Could you check a few things on this model? Use its own coordinates, in mm. A direction names the side the tool comes from. Round coordinates to 2 decimals unless told otherwise and drop trailing zeros. Loops run counter-clockwise (first coordinate to the right, second up) from the corner with the lowest first, then second, coordinate; pieces in that order, holes last. Notation, with made-up numbers: M 7,-11 L 19,-11 A9 ccw 19,6 Z; hole C -15.75,52.25 d1. An arc over 180 degrees is marked long. Answer in a Markdown table with one row per item.
```python
from build123d import *

# Parameters (mm, degrees)
BOSS_EXTRUDE1_DEPTH                 = 7
SKETCH3_W                           = 68
SKETCH3_H                           = 66
BOSS_EXTRUDE2_DEPTH                 = 7
SKETCH5_R                           = 1
HOLE_POSITIONS_DEPTH                = 74.137994469
M5X0_8_TAPPED_HOLE1_D               = 4.2
CBORE_FOR_M3_SHCS1_D                = 3.4
CBORE_FOR_M3_SHCS1_CBORE_D          = 7
CBORE_FOR_M3_SHCS1_CBORE_DEPTH      = 3
FILLET1_R                           = 8
FILLET2_R                           = 4
M3X0_5_TAPPED_HOLE1_D               = 2.5
M3X0_5_TAPPED_HOLE1_DEPTH           = 7.5
M3X0_5_TAPPED_HOLE1_TIP             = 0.751075774
M3X0_5_TAPPED_HOLE1_ON_FACE_2_D     = 2.5
M3X0_5_TAPPED_HOLE1_ON_FACE_2_DEPTH = 7.5
M3X0_5_TAPPED_HOLE1_ON_FACE_2_TIP   = 0.751075774
M3X0_5_TAPPED_HOLE1_ON_FACE_3_D     = 2.5
M3X0_5_TAPPED_HOLE1_ON_FACE_3_DEPTH = 7.5
M3X0_5_TAPPED_HOLE1_ON_FACE_3_TIP   = 0.751075774
CHAMFER1_SIZE                       = 0.8


with BuildPart() as part:
    # Sketch1 → Boss-Extrude1 (new body)
    with BuildSketch(Plane(origin=(0, 0, 0), x_dir=(1, 0, 0), z_dir=(0, 1, 0))):
        Polygon((0, -55.033320997), (47.660254038, 27.516660498), (-47.660254038, 27.516660498), align=None)
    extrude(amount=BOSS_EXTRUDE1_DEPTH)

    # Sketch3 → Boss-Extrude2 (add)
    with BuildSketch(Plane(origin=(0, 0, 0), x_dir=(1, 0, 0), z_dir=(0, 1, 0))):
        with Locations((0, -5.483339502)):
            Rectangle(SKETCH3_W, SKETCH3_H)
    extrude(amount=BOSS_EXTRUDE2_DEPTH)

    # Sketch5 → Hole Positions (cut, through all)
    with BuildSketch(Plane(origin=(0, 7, 0), x_dir=(1, 0, 0), z_dir=(0, 1, 0))):
        with Locations(Location((-34, 19.629909152, 0), (0, 0, 270))):
            Circle(SKETCH5_R)
        with Locations(Location((34, 19.629909152, 0), (0, 0, 270))):
            Circle(SKETCH5_R)
        with Locations(Location((0, -39.259818305, 0), (0, 0, 270))):
            Circle(SKETCH5_R)
    extrude(amount=-HOLE_POSITIONS_DEPTH, mode=Mode.SUBTRACT)

    # M5x0.8 Tapped Hole1 (through all)
    with Locations(Plane(origin=(0, 7, 0), x_dir=(1, 0, 0), z_dir=(0, 1, 0))):
        with Locations((-34, 19.629909152), (34, 19.629909152), (0, -39.259818305)):
            Hole(M5X0_8_TAPPED_HOLE1_D / 2)

    # CBORE for M3 SHCS1 (through all)
    with Locations(Plane(origin=(0, 7, 0), x_dir=(1, 0, 0), z_dir=(0, 1, 0))):
        with Locations((-10, 2), (10, 2), (10, -18), (-10, -18)):
            CounterBoreHole(CBORE_FOR_M3_SHCS1_D / 2, CBORE_FOR_M3_SHCS1_CBORE_D / 2, CBORE_FOR_M3_SHCS1_CBORE_DEPTH)

    # Fillet1
    fillet1_edges = [part.edges().sort_by_distance(p)[0] for p in [
        (-47.660254038, 3.5, -27.516660498),
        (47.660254038, 3.5, -27.516660498),
        (0, 3.5, 55.033320997),
    ]]
    fillet(fillet1_edges, radius=FILLET1_R)

    # Fillet2
    fillet2_edges = [part.edges().sort_by_distance(p)[0] for p in [
        (34, 3.5, -3.856406461),
        (34, 3.5, 38.483339502),
        (-34, 3.5, -3.856406461),
        (-9.555136271, 3.5, 38.483339502),
        (-34, 3.5, 38.483339502),
        (9.555136271, 3.5, 38.483339502),
    ]]
    fillet(fillet2_edges, radius=FILLET2_R)

    # M3x0.5 Tapped Hole1
    with Locations(Plane(origin=(-34, 3.5, 28.483339502), x_dir=(0, 0, -1), z_dir=(-1, 0, 0))):
        with Locations((0, 0)):
            Hole(M3X0_5_TAPPED_HOLE1_D / 2, depth=M3X0_5_TAPPED_HOLE1_DEPTH)
            with Locations((0, 0, -(M3X0_5_TAPPED_HOLE1_DEPTH + M3X0_5_TAPPED_HOLE1_TIP / 2))):  # 118° drill point
                Cone(0, M3X0_5_TAPPED_HOLE1_D / 2, M3X0_5_TAPPED_HOLE1_TIP, mode=Mode.SUBTRACT)

    # M3x0.5 Tapped Hole1 on face 2
    with Locations(Plane(origin=(34, 3.5, 28.483339502), x_dir=(0, 0, 1), z_dir=(1, 0, 0))):
        with Locations((0, 0)):
            Hole(M3X0_5_TAPPED_HOLE1_ON_FACE_2_D / 2, depth=M3X0_5_TAPPED_HOLE1_ON_FACE_2_DEPTH)
            with Locations((0, 0, -(M3X0_5_TAPPED_HOLE1_ON_FACE_2_DEPTH + M3X0_5_TAPPED_HOLE1_ON_FACE_2_TIP / 2))):  # 118° drill point
                Cone(0, M3X0_5_TAPPED_HOLE1_ON_FACE_2_D / 2, M3X0_5_TAPPED_HOLE1_ON_FACE_2_TIP, mode=Mode.SUBTRACT)

    # M3x0.5 Tapped Hole1 on face 3
    with Locations(Plane(origin=(0, 3.5, -27.516660498), x_dir=(-1, 0, 0), z_dir=(0, 0, -1))):
        with Locations((0, 0)):
            Hole(M3X0_5_TAPPED_HOLE1_ON_FACE_3_D / 2, depth=M3X0_5_TAPPED_HOLE1_ON_FACE_3_DEPTH)
            with Locations((0, 0, -(M3X0_5_TAPPED_HOLE1_ON_FACE_3_DEPTH + M3X0_5_TAPPED_HOLE1_ON_FACE_3_TIP / 2))):  # 118° drill point
                Cone(0, M3X0_5_TAPPED_HOLE1_ON_FACE_3_D / 2, M3X0_5_TAPPED_HOLE1_ON_FACE_3_TIP, mode=Mode.SUBTRACT)

    # Chamfer1
    chamfer1_edges = [part.edges().sort_by_distance(p)[0] for p in [
        (-13.5, 7, -2),
        (-8.3, 0, -2),
        (0, 7, -27.516660498),
        (0, 0, -27.516660498),
        (-37.633974596, 0, -10.150635095),
        (7.664319482, 0, 41.758330249),
        (0, 0, 47.033320997),
        (-40.732050808, 0, -23.516660498),
        (40.732050808, 0, -23.516660498),
        (7.664319482, 7, 41.758330249),
        (-37.633974596, 7, -10.150635095),
        (0, 7, 47.033320997),
        (-40.732050808, 7, -23.516660498),
        (40.732050808, 7, -23.516660498),
        (-34, 7, 15.849364905),
        (-34, 0, 15.849364905),
        (-20.932268674, 0, 38.483339502),
        (-20.932268674, 7, 38.483339502),
        (37.633974596, 0, -10.150635095),
        (34, 0, 15.849364905),
        (20.932268674, 0, 38.483339502),
        (-7.664319482, 0, 41.758330249),
        (32.828427125, 0, 37.311766626),
        (-32.828427125, 0, 37.311766626),
        (37.633974596, 7, -10.150635095),
        (-7.664319482, 7, 41.758330249),
        (20.932268674, 7, 38.483339502),
        (34, 7, 15.849364905),
        (32.828427125, 7, 37.311766626),
        (-32.828427125, 7, 37.311766626),
        (-34.136296695, 0, -3.819885871),
        (-34.136296695, 7, -3.819885871),
        (-9.864537348, 7, 39.019237886),
        (-9.864537348, 0, 39.019237886),
        (9.864537348, 0, 39.019237886),
        (9.864537348, 7, 39.019237886),
        (34.136296695, 7, -3.819885871),
        (34.136296695, 0, -3.819885871),
        (2.1, 7, 39.259818305),
        (2.1, 0, 39.259818305),
        (36.1, 7, -19.629909152),
        (36.1, 0, -19.629909152),
        (-31.9, 7, -19.629909152),
        (-31.9, 0, -19.629909152),
        (-13.5, 7, 18),
        (-8.3, 0, 18),
        (6.5, 7, 18),
        (11.7, 0, 18),
        (6.5, 7, -2),
        (11.7, 0, -2),
    ]]
    chamfer(chamfer1_edges, length=CHAMFER1_SIZE)


solid = part.part
```
1) I want a section at C-C, the plane z = 4.5. Please give me the cut outline in (x, y).
Computed:
| item | result |
|---|---|
| outline | M -34,0.8 L -33.2,0 L 33.2,0 L 34,0.8 L 34,6.2 L 33.2,7 L -33.2,7 L -34,6.2 Z |
2) Which directions (+Z, -Z, +X, -X, +Y, -Y) give clear straight access to the entire face, cutting with the end or side of a thin tool? Please do faces 4 (the face through (7.42, 5.115, 15.635)), 5 (the face through (-0.117, 3.538, 47.032)), 6 (the face through (-30.197, 3.979, 29.638)).
Computed:
| item | result |
|---|---|
| face 4 | +Y |
| face 5 | +Z, +Y, -Y |
| face 6 | -X |
3) I want a section at B-B, the plane x = -18. Please give me the cut outline in (y, z), plus the area to 3 significant figures.
Computed:
| item | result |
|---|---|
| outline | M 0,-26.72 L 0.8,-27.52 L 6.2,-27.52 L 7,-26.72 L 7,37.68 L 6.2,38.48 L 0.8,38.48 L 0,37.68 Z |
| area | 461 mm² |
4) I want a section at A-A, the plane z = 18. State how many separate pieces and enclosed holes the cut face has, plus the area to 3 significant figures.
Computed:
| item | result |
|---|---|
| separate pieces | 3 |
| enclosed holes | 0 |
| area | 403 mm² |
5) Will these pins go through, and if not, where does the flat tip stop? P1, Ø1, axis at x = 9, z = -1.5, coming from the +Y side; P2, Ø2, axis at x = -21.5, y = 3, coming from the +Z side; P3, Ø3, axis at y = 3.5, z = 28.48, coming from the -X side; P4, Ø4, axis at y = 3, z = 38, coming from the -X side.
Computed:
| item | result |
|---|---|
| P1 | passes through |
| P2 | stops at z = 38.48 |
| P3 | stops at x = -34 |
| P4 | stops at x = -33.7 |
6) If we mould it in two halves opening along Z, with no side actions, what happens to faces 1 (the face through (-8, 4, 17)), 2 (the face through (34, 3, 16)), 3 (the face through (-9.9, 3.5, 39))? For each: released by +Z, released by -Z, zero draft, split by the parting line, or undercut.
Computed:
| item | result |
|---|---|
| face 1 | undercut |
| face 2 | zero draft |
| face 3 | released by +Z |
7) I need wall thicknesses on line 1 (X direction, y = 5.2, z = 18); line 2 (Y direction, x = 0, z = -22); line 3 (Z direction, x = 11, y = 1.5). Which ranges of each line are inside material? Lowest first, please.
Computed:
| item | result |
|---|---|
| line 1 | x = -34 to -13.5, -6.5 to 6.5, 13.5 to 34 |
| line 2 | y = 0 to 2.25, 4.75 to 7 |
| line 3 | z = -27.52 to -3.37, -0.63 to 16.63, 19.37 to 38.58 |
